Study the drawing (mm; zero at the part's minimum x, y, z) and answer. Round coordinates to 2 decimals unless told otherwise and drop trailing zeros. Order: outer loops, then holes, each group sorted by start corner. A loop starts at its lowest first (then second) coordinate and runs counter-clockwise, first axis right, second up. Notation, with made-up numbers: (-34, -0.75) - (-20, -0.75) arc R11 cw to (-20, 10.25) - close; hole circle Ø6 at (52, 30). An arc over 180 degrees is marked (long way). Put each result on its own line as item: value.
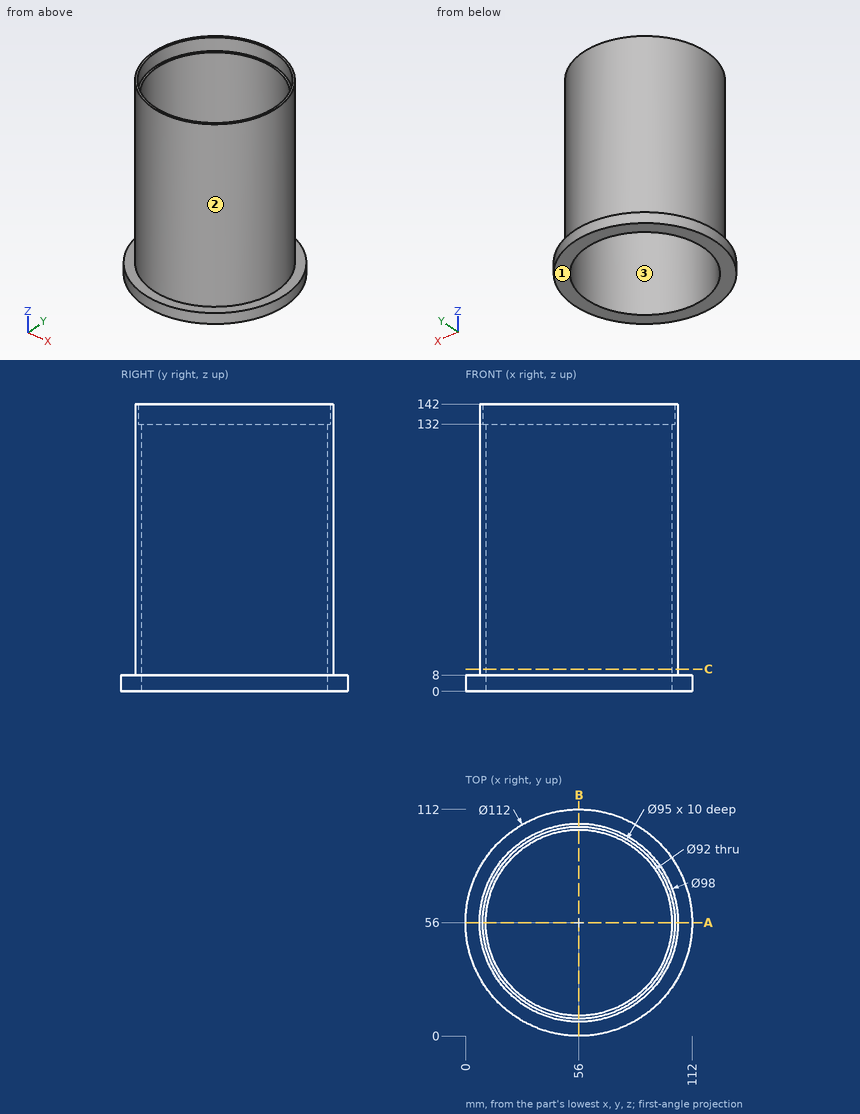
1) A cutting plane is placed at C-C on z = 11. Write down the section's boundary in (x, y).
Findings below:
outline: circle Ø98 at (56, 56); hole circle Ø92 at (56, 56)
2) Straight lines are drawn through the part: L1, parallel to Y at x = 56, z = 84.5; L2, parallel to Y at x = 69, z = 73.5; L3, parallel to X at y = 44, z = 90.5. For each, find the intervals that lie inside material, in ascending order. Write a range as from..to.
Findings below:
L1: y = 7..10, 102..105
L2: y = 8.76..11.88, 100.12..103.24
L3: x = 8.49..11.59, 100.41..103.51
3) For a pull along X with two mould halves and no side action, classify the marked faces 1, 2 and 3 as pulls with the +X half, pulls with the -X half, needs draft (parallel to the pull), parting line crosses it, or undercut.
Findings below:
face 1: needs draft
face 2: parting line crosses it
face 3: undercut
4) A cutting plane is placed at A-A on y = 56. Write down the section's boundary in (x, z), then the cut area to 3 significant figures.
Findings below:
outline: (0, 0) - (10, 0) - (10, 132) - (8.5, 132) - (8.5, 142) - (7, 142) - (7, 8) - (0, 8) - close; (102, 0) - (112, 0) - (112, 8) - (105, 8) - (105, 142) - (103.5, 142) - (103.5, 132) - (102, 132) - close
area: 934 mm2
5) Given pin 1 Ø2 at (y, z) = (30, 126.5) entering from +X; pin 2 Ø10 at (y, z) = (15, 123) entering from -X; pin 3 Ø10 at (y, z) = (60.5, 22.5) entering from -X, each flat-ended and moving along its own axis, determine where each tip first touches the part or whether it passes through.
Findings below:
pin 1: stops at x = 98.14
pin 2: stops at x = 22.76
pin 3: stops at x = 7
